from build123d import *

# Parameters (mm, degrees)
F0_R     = 20.8
F1_DEPTH = 7.75
F2_R     = 2.2
F3_DEPTH = 7.751
F5_DEPTH = 7.751


with BuildPart() as f1:
    # F0 (on Top) → F1 (new body)
    with BuildSketch(Plane.XY):
        Circle(F0_R)
    extrude(amount=F1_DEPTH)

    # F2 (on face) → F3 (cut, through all)
    with BuildSketch(Plane.XY.offset(7.75)):
        with Locations((-5.002671, 12.204482)):
            Circle(F2_R)
        with Locations((-5.002671, 5.104482)):
            Circle(F2_R)
        with Locations((-12.173096, 5.104482)):
            Circle(F2_R)
        with Locations((-12.204482, -5.002671)):
            Circle(F2_R)
        with Locations((-5.104482, -5.002671)):
            Circle(F2_R)
        with Locations((-5.104482, -12.173096)):
            Circle(F2_R)
        with Locations((5.002671, -12.204482)):
            Circle(F2_R)
        with Locations((5.002671, -5.104482)):
            Circle(F2_R)
        with Locations((12.173096, -5.104482)):
            Circle(F2_R)
        with Locations((12.204482, 5.002671)):
            Circle(F2_R)
        with Locations((5.104482, 5.002671)):
            Circle(F2_R)
        with Locations((5.104482, 12.173096)):
            Circle(F2_R)
    extrude(amount=-F3_DEPTH, mode=Mode.SUBTRACT)

    # F4 (on face) → F5 (cut, through all)
    with BuildSketch(Plane(origin=(0, 0, 0), x_dir=(1, 0, 0), z_dir=(0, 0, -1))):
        with BuildLine():
            Line((6.799199, 0.6), (6.799199, -0.6))
            Line((6.799199, -0.6), (7.999199, -0.6))
            Line((7.999199, -0.6), (7.999199, -1.8))
            Line((7.999199, -1.8), (7.999199, -5.344601))
            ThreePointArc((7.999199, -5.344601), (8.5996, -5.945002), (9.2, -5.344601))
            Line((9.2, -5.344601), (9.2, -1.8))
            Line((9.2, -1.8), (9.2, -0.6))
            Line((9.2, -0.6), (10.4, -0.6))
            Line((10.4, -0.6), (10.4, 0.6))
            Line((10.4, 0.6), (9.2, 0.6))
            Line((9.2, 0.6), (9.2, 1.8))
            Line((9.2, 1.8), (9.2, 5.3))
            ThreePointArc((9.2, 5.3), (8.5996, 5.9004), (7.999199, 5.3))
            Line((7.999199, 5.3), (7.999199, 1.8))
            Line((7.999199, 1.8), (7.999199, 0.6))
            Line((7.999199, 0.6), (6.799199, 0.6))
        make_face()
        with BuildLine():
            Line((-1.8, 9.2), (-5.3, 9.2))
            ThreePointArc((-5.3, 9.2), (-5.9004, 8.5996), (-5.3, 7.999199))
            Line((-5.3, 7.999199), (-1.8, 7.999199))
            Line((-1.8, 7.999199), (-0.6, 7.999199))
            Line((-0.6, 7.999199), (-0.6, 6.799199))
            Line((-0.6, 6.799199), (0.6, 6.799199))
            Line((0.6, 6.799199), (0.6, 7.999199))
            Line((0.6, 7.999199), (1.8, 7.999199))
            Line((1.8, 7.999199), (5.344601, 7.999199))
            ThreePointArc((5.344601, 7.999199), (5.945002, 8.5996), (5.344601, 9.2))
            Line((5.344601, 9.2), (1.8, 9.2))
            Line((1.8, 9.2), (0.6, 9.2))
            Line((0.6, 9.2), (0.6, 10.4))
            Line((0.6, 10.4), (-0.6, 10.4))
            Line((-0.6, 10.4), (-0.6, 9.2))
            Line((-0.6, 9.2), (-1.8, 9.2))
        make_face()
        with BuildLine():
            Line((-9.2, -1.8), (-9.2, -5.3))
            ThreePointArc((-9.2, -5.3), (-8.5996, -5.9004), (-7.999199, -5.3))
            Line((-7.999199, -5.3), (-7.999199, -1.8))
            Line((-7.999199, -1.8), (-7.999199, -0.6))
            Line((-7.999199, -0.6), (-6.799199, -0.6))
            Line((-6.799199, -0.6), (-6.799199, 0.6))
            Line((-6.799199, 0.6), (-7.999199, 0.6))
            Line((-7.999199, 0.6), (-7.999199, 1.8))
            Line((-7.999199, 1.8), (-7.999199, 5.344601))
            ThreePointArc((-7.999199, 5.344601), (-8.5996, 5.945002), (-9.2, 5.344601))
            Line((-9.2, 5.344601), (-9.2, 1.8))
            Line((-9.2, 1.8), (-9.2, 0.6))
            Line((-9.2, 0.6), (-10.4, 0.6))
            Line((-10.4, 0.6), (-10.4, -0.6))
            Line((-10.4, -0.6), (-9.2, -0.6))
            Line((-9.2, -0.6), (-9.2, -1.8))
        make_face()
        with BuildLine():
            Line((1.8, -9.2), (5.3, -9.2))
            ThreePointArc((5.3, -9.2), (5.9004, -8.5996), (5.3, -7.999199))
            Line((5.3, -7.999199), (1.8, -7.999199))
            Line((1.8, -7.999199), (0.6, -7.999199))
            Line((0.6, -7.999199), (0.6, -6.799199))
            Line((0.6, -6.799199), (-0.6, -6.799199))
            Line((-0.6, -6.799199), (-0.6, -7.999199))
            Line((-0.6, -7.999199), (-1.8, -7.999199))
            Line((-1.8, -7.999199), (-5.344601, -7.999199))
            ThreePointArc((-5.344601, -7.999199), (-5.945002, -8.5996), (-5.344601, -9.2))
            Line((-5.344601, -9.2), (-1.8, -9.2))
            Line((-1.8, -9.2), (-0.6, -9.2))
            Line((-0.6, -9.2), (-0.6, -10.4))
            Line((-0.6, -10.4), (0.6, -10.4))
            Line((0.6, -10.4), (0.6, -9.2))
            Line((0.6, -9.2), (1.8, -9.2))
        make_face()
    extrude(amount=-F5_DEPTH, mode=Mode.SUBTRACT)


solid = f1.part
Geometry check sheet. Reference: the model listing, model coordinates, mm. Give positions to 0.01 mm unless a question says otherwise; leave off trailing zeros. Order: outer loops, then holes, each group sorted by start corner. A loop starts at its lowest first (then second) coordinate and runs counter-clockwise, first axis right, second up. Notation, with made-up numbers: (-3, 87.25) - (31, 87.25) arc R25 cw to (31, 107.25) - close; hole circle Ø1 at (24, 13.25). An arc over 180 degrees is marked (long way). Answer as a JSON object with one key per item and string values.
(1) Draft check along X on faces 1 (the cylindrical face through (-2.708, 20.623, 3.821)), 2 (the flat face through (9.2, 3, 4)). Enter one of: released by +X, released by -X, zero draft, split by the parting line, or undercut.
Report:
{"face 1": "split by the parting line", "face 2": "undercut"}
(2) Cross-section at D-D (z = 5.75). State how many separate pieces and enclosed holes the cut face has, then the cut area to 3 significant figures.
Report:
{"separate pieces": "1", "enclosed holes": "16", "area": "1,110 mm^2"}
(3) Cross-section at A-A (y = 0). Record the cut outline in (x, z).
Report:
{"outline": "(-20.8, 0) - (-10.4, 0) - (-10.4, 7.75) - (-20.8, 7.75) - close; (-6.8, 0) - (6.8, 0) - (6.8, 7.75) - (-6.8, 7.75) - close; (10.4, 0) - (20.8, 0) - (20.8, 7.75) - (10.4, 7.75) - close"}
(4) Material ranges on line 1 (Y direction, x = 11, z = 7.25); line 2 (X direction, y = -12, z = 3); line 3 (Y direction, x = -6, z = 1), recorded low to high.
Report:
{"line 1": "-17.65 to -6.97, -3.24 to 3.16, 6.84 to 17.65", "line 2": "-16.99 to -7.3, -2.91 to 2.81, 7.19 to 16.99", "line 3": "-19.92 to -14.18, -10.16 to -7.01, -2.99 to 3.14, 7.07 to 10.24, 14.17 to 19.92"}
(5) Cross-section at C-C (x = -18). Record the cut outline in (y, z), then the cut area to 3 significant figures.
Report:
{"outline": "(-10.42, 0) - (10.42, 0) - (10.42, 7.75) - (-10.42, 7.75) - close", "area": "162 mm^2"}
(6) Cross-section at B-B (x = 4). Record the cut outline in (y, z).
Report:
{"outline": "(-20.41, 0) - (-14.16, 0) - (-14.16, 7.75) - (-20.41, 7.75) - close; (-10.25, 0) - (-9.2, 0) - (-9.2, 7.75) - (-10.25, 7.75) - close; (-8, 0) - (-7.06, 0) - (-7.06, 7.75) - (-8, 7.75) - close; (-3.15, 0) - (3.1, 0) - (3.1, 7.75) - (-3.15, 7.75) - close; (6.91, 0) - (8, 0) - (8, 7.75) - (6.91, 7.75) - close; (9.2, 0) - (10.27, 0) - (10.27, 7.75) - (9.2, 7.75) - close; (14.08, 0) - (20.41, 0) - (20.41, 7.75) - (14.08, 7.75) - close"}
(7) Depth check by flat-ended pin: pin 1 Ø1.5 at (y, z) = (-5.5, 2.5) entering from +X; pin 2 Ø2 at (x, z) = (-12, 1) entering from -Y; pin 3 Ø1 at (x, z) = (13, 3.5) entering from -Y (3 decimals); pin 4 Ø4 at (x, y) = (-12.17, 5.1) entering from +Z. Enter the tip coordinate at first touch or a pass-through.
Report:
{"pin 1": "x = 20.25", "pin 2": "y = -17.65", "pin 3": "y = -16.625", "pin 4": "through"}
